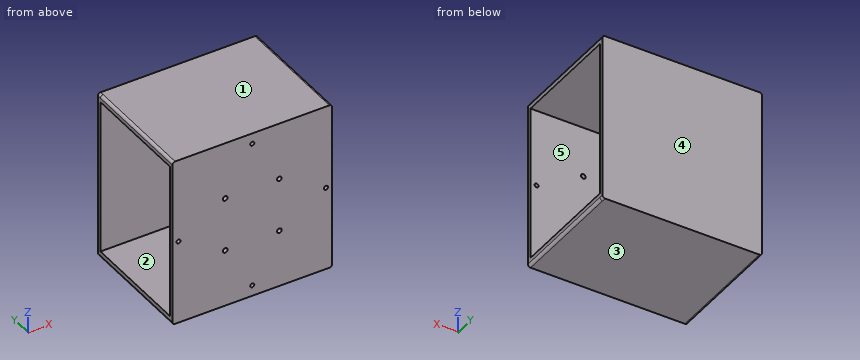
from build123d import *

# Parameters (mm, degrees)
SKETCH_1_W          = 118
SKETCH_1_H          = 125
SKETCH_1_R          = 1.5
EXTRUDE_1_DEPTH     = 3
SKETCH_5_R          = 1.75
CUT_EXTRUDE_1_DEPTH = 10
SKETCH_6_W          = 118
SKETCH_6_H          = 5
EXTRUDE_4_DEPTH     = 82
FILLET_1_R          = 2
SKETCH_7_W          = 118
SKETCH_7_H          = 125
EXTRUDE_5_DEPTH     = 3
FILLET_2_R          = 2


with BuildPart() as part:
    # 草图1 → 凸台-拉伸1 (new body)
    with BuildSketch(Plane(origin=(0, 0, 0), x_dir=(1, 0, 0), z_dir=(0, 1, 0))):
        Rectangle(SKETCH_1_W, SKETCH_1_H)
        with Locations(Location((-54.5, 0, 0), (0, 0, 270))):
            Circle(SKETCH_1_R, mode=Mode.SUBTRACT)
        with Locations(Location((0, 54.5, 0), (0, 0, 270))):
            Circle(SKETCH_1_R, mode=Mode.SUBTRACT)
        with Locations(Location((54.5, 0, 0), (0, 0, 270))):
            Circle(SKETCH_1_R, mode=Mode.SUBTRACT)
        with Locations(Location((0, -54.5, 0), (0, 0, 270))):
            Circle(SKETCH_1_R, mode=Mode.SUBTRACT)
    extrude(amount=EXTRUDE_1_DEPTH)

    # 草图5 → 切除-拉伸1 (cut)
    with BuildSketch(Plane(origin=(0, 0, 0), x_dir=(-1, 0, 0), z_dir=(0, -1, 0))):
        with Locations(Location((20, 20, 0), (0, 0, 90))):
            Circle(SKETCH_5_R)
        with Locations(Location((-20, 20, 0), (0, 0, 90))):
            Circle(SKETCH_5_R)
        with Locations(Location((-20, -20, 0), (0, 0, 90))):
            Circle(SKETCH_5_R)
        with Locations(Location((20, -20, 0), (0, 0, 90))):
            Circle(SKETCH_5_R)
    extrude(amount=-CUT_EXTRUDE_1_DEPTH, mode=Mode.SUBTRACT)

    # 草图6 → 凸台-拉伸4 (add)
    with BuildSketch(Plane(origin=(0, 3, 0), x_dir=(1, 0, 0), z_dir=(0, 1, 0))):
        with Locations((0, -60)):
            Rectangle(SKETCH_6_W, SKETCH_6_H)
        with Locations((0, 60)):
            Rectangle(SKETCH_6_W, SKETCH_6_H)
    extrude(amount=EXTRUDE_4_DEPTH)

    # 圆角1
    fillet_1_edges = [part.edges().sort_by_distance(p)[0] for p in [
        (-59, 42.5, -62.5),
        (59, 42.5, -62.5),
        (59, 42.5, 62.5),
        (-59, 42.5, 62.5),
    ]]
    fillet(fillet_1_edges, radius=FILLET_1_R)

    # 草图7 → 凸台-拉伸5 (add)
    with BuildSketch(Plane(origin=(0, 85, 0), x_dir=(1, 0, 0), z_dir=(0, 1, 0))):
        Rectangle(SKETCH_7_W, SKETCH_7_H)
    extrude(amount=EXTRUDE_5_DEPTH)

    # 圆角2
    fillet_2_edges = [part.edges().sort_by_distance(p)[0] for p in [
        (-59, 86.5, -62.5),
        (59, 86.5, -62.5),
        (-59, 86.5, 62.5),
        (59, 86.5, 62.5),
    ]]
    fillet(fillet_2_edges, radius=FILLET_2_R)


solid = part.part
Can you work these out from the model? Positions are in its coordinate system, mm. Face numbers are marked on the shaded views. A direction names the side the tool comes from. Coordinates: 2 decimals unless noted, no trailing zeros. Write each loop counter-clockwise with the first axis right and the second up, starting at its lowest first coordinate (ties: lowest second). Pieces come first, ordered by that corner, then holes. Notation, with made-up numbers: (42.25, 14) -> (83.25, 14) arc R24 ccw to (83.25, 28) -> close; hole circle Ø4 at (5.5, 84.5). An arc over 180 degrees is marked (long way). Write item = value, one per line.
(1) Imagine slicing it at C-C (z = 20). Please give me the cut outline in (x, y), and give its area (3 significant figures).
Verdict:
outline = (-59, 0) -> (-21.75, 0) -> (-21.75, 3) -> (-59, 3) -> close; (-59, 85) -> (59, 85) -> (59, 88) -> (-59, 88) -> close; (-18.25, 0) -> (18.25, 0) -> (18.25, 3) -> (-18.25, 3) -> close; (21.75, 0) -> (59, 0) -> (59, 3) -> (21.75, 3) -> close
area = 687 mm^2
(2) If I drill on probe 1 along X at (y, z) = (1.5, 0); probe 2 along X at (y, z) = (1.05, 20); probe 3 along X at (y, z) = (1.6, 54.5), over which ranges is the centre line in solid material (lowest first)?
Verdict:
probe_1 = -59 to -56, -53 to 53, 56 to 59
probe_2 = -59 to -21.75, -18.25 to 18.25, 21.75 to 59
probe_3 = -59 to -1.5, 1.5 to 59
(3) Thinking about a two-plate mould opening in Y: for the marked faces 3, 4 and 5, which applies, +Y half, -Y half, draft (parallel to the pull), parting line (faces both ways), or undercut?
Verdict:
face_3 = draft
face_4 = +Y half
face_5 = undercut
(4) Imagine slicing it at A-A (y = 16). Please give me the cut outline in (x, z), and give its area (3 significant figures).
Verdict:
outline = (-59, -60.5) arc R2 ccw to (-57, -62.5) -> (57, -62.5) arc R2 ccw to (59, -60.5) -> (59, -57.5) -> (-59, -57.5) -> close; (-59, 57.5) -> (59, 57.5) -> (59, 60.5) arc R2 ccw to (57, 62.5) -> (-57, 62.5) arc R2 ccw to (-59, 60.5) -> close
area = 1,180 mm^2
(5) Imagine slicing it at B-B (x = -20). Please give me the cut outline in (y, z).
Verdict:
outline = (0, -62.5) -> (88, -62.5) -> (88, 62.5) -> (0, 62.5) -> (0, 21.75) -> (3, 21.75) -> (3, 57.5) -> (85, 57.5) -> (85, -57.5) -> (3, -57.5) -> (3, -21.75) -> (0, -21.75) -> close; (0, -18.25) -> (3, -18.25) -> (3, 18.25) -> (0, 18.25) -> close
(6) Imagine slicing it at D-D (z = -34). Please give me the cut outline in (x, y).
Verdict:
outline = (-59, 0) -> (59, 0) -> (59, 3) -> (-59, 3) -> close; (-59, 85) -> (59, 85) -> (59, 88) -> (-59, 88) -> close
(7) On a 3-axis mill with a long thin cutter (end or side, diameter ignored), from which of +Z, -Z, +X, -X, +Y, -Y can I reach the whole of each face in a straight line? I mean the marked faces 1 and 2. Say none if no direction works.
Verdict:
face_1 = +Z, +X, -X, +Y, -Y
face_2 = +X, -X
(8) For pin 1 (1 mm diameter, centred on x = 58.5, z = 62, fed in from -Y), with a flat end and sliding along its axis, tell me the tip position at first contact or that it passes through.
Verdict:
pin_1 = 0
